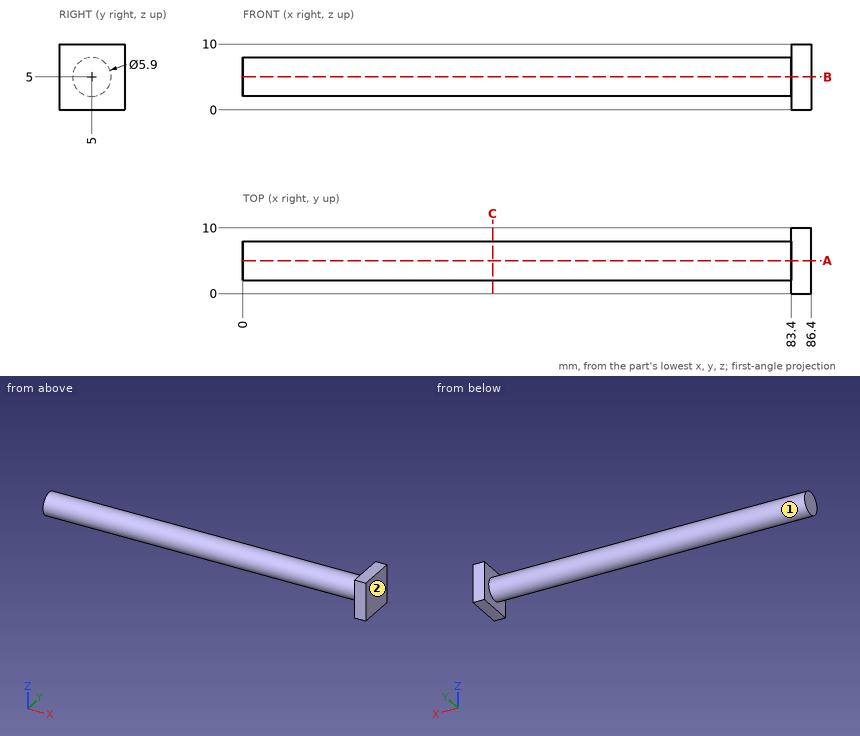
For this review, use the dimensioned drawing (mm, ordinates from the lowest corner) and the shaded views. Give positions to 0.01 mm unless a question says otherwise; leave off trailing zeros. Order: outer loops, then holes, each group sorted by start corner. A loop starts at its lowest first (then second) coordinate and runs counter-clockwise, first axis right, second up. Notation, with made-up numbers: (27.25, 43.5) - (70.25, 43.5) arc R16 ccw to (70.25, 50.5) - close; hole circle Ø7 at (-28, 83). An arc over 180 degrees is marked (long way). Use CSV: the item, a comma, the result in double quotes. Start each with the question number.
Q1. Take a section at C-C (x = 38). State the section outline as (y, z) points, and give its area (3 significant figures).
Q2. For line 1 (X direction, y = 7, z = 2); line 2 (Y direction, x = 65, z = 5); line 3 (Y direction, x = 47, z = 7.25), list the stretches that pass through material, from the lowest coordinate up.
Q3. For P1, Ø6, axis at x = 77.5, z = 7.5, coming from the -Y side; P2, Ø3, axis at x = 35, y = 5, coming from the -Z side, all flat-tipped, find the tip position at first contact; note any pin that passes through.
Q4. Take a section at A-A (y = 5). State the section outline as (x, z) points, and give its area (3 significant figures).
Q5. Draft analysis for pull direction X (two halves, no side actions). For the marked faces 1 and 2, state which applies: pulls with the +X half, pulls with the -X half, needs draft (parallel to the pull), parting line crosses it, or undercut.
Calculated:
1,outline,"circle Ø5.9 at (5, 5)"
1,area,"27.3 mm²"
2,line 1,"x = 83.4 to 86.4"
2,line 2,"y = 2.05 to 7.95"
2,line 3,"y = 3.09 to 6.91"
3,P1,"stops at y = 2.05"
3,P2,"stops at z = 2.05"
4,outline,"(0, 2.05) - (83.4, 2.05) - (83.4, 0) - (86.4, 0) - (86.4, 10) - (83.4, 10) - (83.4, 7.95) - (0, 7.95) - close"
4,area,"522 mm²"
5,face 1,"needs draft"
5,face 2,"pulls with the +X half"
